Geometry check sheet. Reference: the model listing, model coordinates, mm. A direction names the side the tool comes from. Coordinates: 2 decimals unless noted, no trailing zeros. Loops run counter-clockwise (first coordinate to the right, second up) from the corner with the lowest first, then second, coordinate; pieces in that order, holes last.
Autodesk Inventor part; units mm, degrees
ref_plane "YZ Plane" through (0, 0, 0) normal (1, 0, 0) x (0, 1, 0)
ref_plane "XZ Plane" through (0, 0, 0) normal (0, 1, 0) x (-1, 0, 0)
ref_plane "XY Plane" through (0, 0, 0) normal (0, 0, 1) x (1, 0, 0)
sketch "Sketch1" plane through (0, 0, 0) normal (0, 0, 1) x (1, 0, 0)
  circle A0 centre (-17.1376, -0.8341) radius 15.875
  circle A1 centre (-17.1376, -9.7932) radius 1.5875
  circle A2 centre (-8.1786, -0.8341) radius 1.5875
  circle A3 centre (-17.1376, 8.1249) radius 1.5875
  circle A4 centre (-26.0966, -0.8341) radius 1.5875
  line L0 (-19.6376, -0.8341) -> (-15.1013, -2.2845)
  arc A5 (-15.1013, -2.2845) -> (-19.6376, -0.8341) centre (-17.1376, -0.8341) ccw
  arc A6 (-15.1013, -2.2845) -> (-19.6376, -0.8341) centre (-17.1376, -0.8341) ccw
  arc A7 (-15.1013, -2.2845) -> (-19.6376, -0.8341) centre (-17.1376, -0.8341) ccw
  point P0 (0, 0)
  dimension "d0" = 5
  dimension "d1" = 31.75
  dimension "d2" = 3.175
  dimension "d5" = 360
extrude "Extrusion1" add sketch "Sketch1" along normal blind 6.35 contours A0 | A5 L0
sketch "Sketch2" plane through (-17.1376, -0.8341, 0) normal (0, 0, -1) x (-1, 0, 0)
  line L0 (2.5, 0) -> (-2.0363, -1.4504)
  arc A0 (2.5, 0) -> (-2.0363, -1.4504) centre (0, 0) ccw
  point P0 (-17.1376, 0.8341)
extrude "Extrusion2" cut sketch "Sketch2" against normal through all
properties part number "stepperShaftCollar"
(1) Gauge pin test, flat ends, axial feed: pin 1 Ø4 at (x, y) = (-17.14, -9.79) entering from +Z; pin 2 Ø2 at (y, z) = (6.5, 3) entering from +X; pin 3 Ø2 at (x, z) = (-10, 3.5) entering from -Y; pin 4 Ø3 at (y, z) = (11.5, 4) entering from -X. Record the tip position at first contact, or that the pin passes through.
Findings:
pin 1: stops at z = 6.35
pin 2: stops at x = -2.58
pin 3: stops at y = -15.47
pin 4: stops at x = -28.74
(2) Draft check along X on faces 1 (the flat face through (-17, -4, 0)), 2 (the cylindrical face through (-33, -1.5, 3.1)), 3 (the cylindrical face through (-16.439, 1.566, 3.131)). Enter one of: +X half, -X half, draft (parallel to the pull), parting line (faces both ways), or undercut.
Findings:
face 1: draft
face 2: parting line
face 3: undercut
(3) Sectioned sample at C-C on x = -17.5. Record the cut outline in (y, z), and give its area (3 significant figures).
Findings:
outline: (-16.7, 0) - (-11.34, 0) - (-11.34, 6.35) - (-16.7, 6.35) - close; (-8.25, 0) - (-1.52, 0) - (-1.52, 6.35) - (-8.25, 6.35) - close; (1.64, 0) - (6.58, 0) - (6.58, 6.35) - (1.64, 6.35) - close; (9.67, 0) - (15.04, 0) - (15.04, 6.35) - (9.67, 6.35) - close
area: 142 mm2
(4) Scan lines: L1, parallel to Y at x = -16, z = 1.25; L2, parallel to X at y = 8, z = 4; L3, parallel to Y at x = -8, z = 1. Record each from-to range of solid material in increasing order.
Findings:
L1: y = -16.67 to -10.9, -8.69 to -2, 1.39 to 7.02, 9.23 to 15
L2: x = -30.33 to -18.72, -15.56 to -3.95
L3: y = -13.82 to -2.41, 0.74 to 12.15
(5) Sectioned sample at A-A on y = -11. Record the cut outline in (x, z).
Findings:
outline: (-29.33, 0) - (-18.17, 0) - (-18.17, 6.35) - (-29.33, 6.35) - close; (-16.11, 0) - (-4.94, 0) - (-4.94, 6.35) - (-16.11, 6.35) - close
(6) Sectioned sample at B-B on x = -9. Record the cut outline in (y, z), and give its area (3 significant figures).
Findings:
outline: (-14.46, 0) - (-2.19, 0) - (-2.19, 6.35) - (-14.46, 6.35) - close; (0.52, 0) - (12.8, 0) - (12.8, 6.35) - (0.52, 6.35) - close
area: 156 mm2
(7) Sectioned sample at D-D on z = 1.75. State how many separate pieces and enclosed holes the cut face has, and give its area (3 significant figures).
Findings:
separate pieces: 1
enclosed holes: 5
area: 746 mm2
(8) Access from +Z, -Z, +X, -X, +Y, -Y to the whole of each face (thin tool, end or side, straight path). Record for faces 4 (the flat face through (-17, -4, 6.35)), 5 (the flat face through (-17.4, -1.55, 3.13)).
Findings:
face 4: +Z, +X, -X, +Y, -Y
face 5: +Z, -Z
